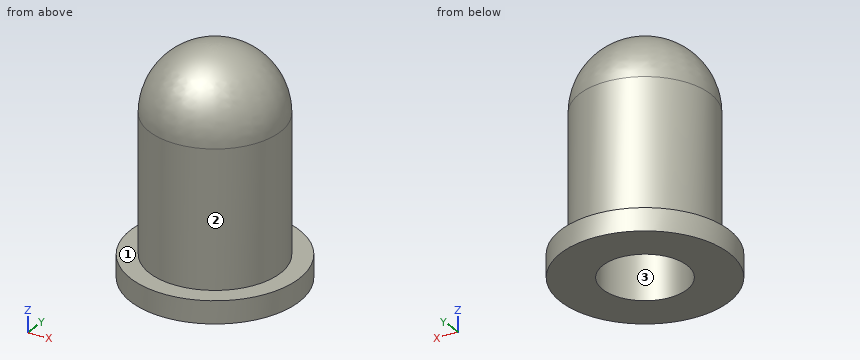
from build123d import *


with BuildPart() as f1:
    # F0 (on Front) → F1 (revolve)
    with BuildSketch(Plane.XZ):
        with BuildLine():
            Line((-4.5, 1.2), (-4.5, 0))
            Line((-4.5, 0), (-2.25, 0))
            Line((-2.25, 0), (-2.25, 6.670383))
            ThreePointArc((-2.25, 6.670383), (-2.618768, 9.745815), (0, 11.4))
            Line((0, 11.4), (0, 12))
            ThreePointArc((0, 12), (-2.474874, 10.974874), (-3.5, 8.5))
            Line((-3.5, 8.5), (-3.5, 1.2))
            Line((-3.5, 1.2), (-4.5, 1.2))
        make_face()
    revolve(axis=Axis((0, 0, 11.7), (0, 0, -1)))


solid = f1.part
Source: CAD feature listing. Evaluate the final solid. Frame: model axes, mm. Face numbers are marked on the shaded views. Give positions to 0.01 mm unless a question says otherwise; leave off trailing zeros. Order: outer loops, then holes, each group sorted by start corner. A loop starts at its lowest first (then second) coordinate and runs counter-clockwise, first axis right, second up. Notation, with made-up numbers: (-1, -28) -> (28, -28) arc R29 cw to (28, 9) -> close; hole circle Ø10 at (-17.5, 79). An arc over 180 degrees is marked (long way). Write item = value, one per line.
Item 1: Section query C-C (x = 3.75). Output: boundary loops of the cut face in (y, z), then the cut area to 3 significant figures.
Check result:
outline = (-2.49, 0) -> (2.49, 0) -> (2.49, 1.2) -> (-2.49, 1.2) -> close
area = 5.97 mm²
Item 2: Mould query, pull axis X, two halves, no side actions, for the marked faces 1, 2 and 3. Classes: +X half, -X half, draft (parallel to the pull), parting line (faces both ways), or undercut.
Check result:
face_1 = draft
face_2 = parting line
face_3 = undercut
Item 3: Section query B-B (y = 4.25). Output: boundary loops of the cut face in (x, z).
Check result:
outline = (-1.48, 0) -> (1.48, 0) -> (1.48, 1.2) -> (-1.48, 1.2) -> close
Item 4: Contact query for flat-ended pins moving along their axis: pin 1 (1 mm diameter, centred on x = -2, z = 9.5, fed in from +Y); pin 2 (3 mm diameter, centred on y = -2, z = 8, fed in from -X); pin 3 (2 mm diameter, centred on x = -2, z = 3, fed in from +Y). Output: stop coordinate, or through.
Check result:
pin_1 = 3.04
pin_2 = -3.46
pin_3 = 3.35
Item 5: Ray query, probe 1 along Y at (x, z) = (0, 2.25); probe 2 along X at (y, z) = (-0.75, 9); probe 3 along Y at (x, z) = (-1, 10.5). Return the intervals inside material, ascending.
Check result:
probe_1 = -3.5 to -2.25, 2.25 to 3.5
probe_2 = -3.38 to -2.76, 2.76 to 3.38
probe_3 = -2.69 to -1.85, 1.85 to 2.69
Item 6: Section query A-A (z = 3.5). Output: boundary loops of the cut face in (x, y), then the cut area to 3 significant figures.
Check result:
outline = circle Ø7 at (0, 0); hole circle Ø4.5 at (0, 0)
area = 22.6 mm²
